```python
from build123d import *

# Parameters (mm, degrees)
F1_W     = 12
F1_H     = 14
F1_R     = 2.6
F2_DEPTH = 6
F3_DEPTH = 50
F4_R     = 11.5
F4_R_2   = 1.6
F5_DEPTH = 20.001
F7_R     = 5
F8_SIZE  = 2.5


with BuildPart() as f2:
    # F1 (on Top) → F2 (new body)
    with BuildSketch(Plane.XY):
        with Locations((-10, 30.4999971617)):
            Rectangle(F1_W, F1_H)
        with Locations((-10, 30.4999971617)):
            Circle(F1_R, mode=Mode.SUBTRACT)
        with BuildLine():
            Line((10, 33.0999971617), (10, 37.4999971617))
            Line((10, 37.4999971617), (4, 37.4999971617))
            Line((4, 37.4999971617), (4, 30.4999971617))
            Line((4, 30.4999971617), (7.4, 30.4999971617))
            ThreePointArc((7.4, 30.4999971617), (8.1615223689, 32.3384747928), (10, 33.0999971617))
        make_face()
        with BuildLine():
            Line((16, 30.4999971617), (16, 37.4999971617))
            Line((16, 37.4999971617), (10, 37.4999971617))
            Line((10, 37.4999971617), (10, 33.0999971617))
            ThreePointArc((10, 33.0999971617), (11.8384776311, 32.3384747928), (12.6, 30.4999971617))
            Line((12.6, 30.4999971617), (16, 30.4999971617))
        make_face()
        with BuildLine():
            Line((10, 23.4999971617), (16, 23.4999971617))
            Line((16, 23.4999971617), (16, 30.4999971617))
            Line((16, 30.4999971617), (12.6, 30.4999971617))
            ThreePointArc((12.6, 30.4999971617), (11.8384776311, 28.6615195306), (10, 27.8999971617))
            Line((10, 27.8999971617), (10, 23.4999971617))
        make_face()
        with BuildLine():
            Line((4, 23.4999971617), (10, 23.4999971617))
            Line((10, 23.4999971617), (10, 27.8999971617))
            ThreePointArc((10, 27.8999971617), (8.1615223689, 28.6615195306), (7.4, 30.4999971617))
            Line((7.4, 30.4999971617), (4, 30.4999971617))
            Line((4, 30.4999971617), (4, 23.4999971617))
        make_face()
        Polygon((-16, 37.4999971617), (-20, 23.4999971617), (-16, 23.4999971617), align=None)
        Polygon((-4, 37.4999971617), (-4, 23.4999971617), (4, 23.4999971617), (4, 30.4999971617), (4, 37.4999971617), align=None)
        Polygon((16, 23.4999971617), (20, 23.4999971617), (16, 37.4999971617), (16, 30.4999971617), align=None)
    extrude(amount=F2_DEPTH)

    # F1 (on Top) → F3 (join)
    with BuildSketch(Plane.XY):
        Polygon((-20, 23.4999971617), (-20, 17.4999971617), (20, 17.4999971617), (20, 23.4999971617), (16, 23.4999971617), (10, 23.4999971617), (4, 23.4999971617), (-4, 23.4999971617), (-16, 23.4999971617), align=None)
    extrude(amount=F3_DEPTH)

    # F4 (on face) → F5 (cut, through all)
    with BuildSketch(Plane.XZ.offset(-17.4999971617)):
        with Locations((0, 30)):
            Circle(F4_R)
        with Locations((-15.5, 45.5)):
            Circle(F4_R_2)
        with Locations((-15.5, 14.5)):
            Circle(F4_R_2)
        with Locations((15.5, 14.5)):
            Circle(F4_R_2)
        with Locations((15.5, 45.5)):
            Circle(F4_R_2)
    extrude(amount=-F5_DEPTH, mode=Mode.SUBTRACT)

    # F7
    f7_edges = [f2.edges().sort_by_distance(p)[0] for p in [
        (16, 37.499997, 3),
        (-16, 37.499997, 3),
    ]]
    fillet(f7_edges, radius=F7_R)

    # F8
    f8_edges = [f2.edges().sort_by_distance(p)[0] for p in [
        (-11.5, 23.499997, 30),
    ]]
    chamfer(f8_edges, length=F8_SIZE)


solid = f2.part
```
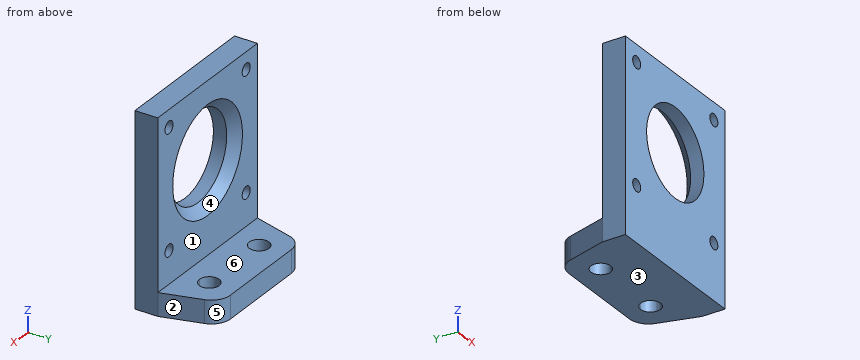
For this review, take the finished solid that the model builds, in its own axes (mm). Face numbers are marked on the shaded views. A direction names the side the tool comes from. Round coordinates to 2 decimals unless told otherwise and drop trailing zeros. Write each loop counter-clockwise with the first axis right and the second up, starting at its lowest first coordinate (ties: lowest second). Pieces come first, ordered by that corner, then holes. Notation, with made-up numbers: (-7, 42) - (16, 42) arc R28 ccw to (16, 70) - close; hole circle Ø7 at (53.25, 52). An arc over 180 degrees is marked (long way). Answer as a JSON object with one key per item and string values.
1. We need section D-D on z = 9.5. Give the boundary of the cut face in (x, y), then the cut area to 3 significant figures.
Response values:
{"outline": "(-20, 17.5) - (20, 17.5) - (20, 23.5) - (-20, 23.5) - close", "area": "240 mm2"}
2. Draft analysis for pull direction Z (two halves, no side actions). For the marked faces 3, 4, 5 and 6, state which applies: +Z half, -Z half, draft (parallel to the pull), parting line (faces both ways), or undercut.
Response values:
{"face 3": "-Z half", "face 4": "undercut", "face 5": "draft", "face 6": "+Z half"}
3. For pin 1 Ø5 at (x, y) = (-7, 21.5) entering from -Z; pin 2 Ø1.5 at (x, y) = (-5, 27.5) entering from +Z; pin 3 Ø3 at (x, z) = (13.5, 40) entering from +Y, all flat-tipped, find the tip position at first contact; note any pin that passes through.
Response values:
{"pin 1": "stops at z = 0", "pin 2": "stops at z = 6", "pin 3": "stops at y = 23.5"}
4. We need section B-B on y = 31.25. Give the boundary of the cut face in (x, z), then the cut area to 3 significant figures.
Response values:
{"outline": "(-17.79, 0) - (-12.49, 0) - (-12.49, 6) - (-17.79, 6) - close; (-7.51, 0) - (7.51, 0) - (7.51, 6) - (-7.51, 6) - close; (12.49, 0) - (17.79, 0) - (17.79, 6) - (12.49, 6) - close", "area": "154 mm2"}
5. Tool access review of the marked faces 1 and 2: name each direction out of +Z, -Z, +X, -X, +Y, -Y from which nothing blocks a thin tool from reaching the whole face with its end or side.
Response values:
{"face 1": "+Z, +X, -X, +Y", "face 2": "+Z, -Z, +X, +Y"}
6. To check wall thickness, follow line 1 along Z through (x, y) = (-15.5, 21.85); line 2 along Z through (x, y) = (16.5, 18.5); line 3 along Z through (x, y) = (0, 18.3). State the ranges of each line that lie inside material, in increasing order.
Response values:
{"line 1": "z = 0 to 12.9, 16.1 to 43.9, 47.1 to 50", "line 2": "z = 0 to 13.25, 15.75 to 44.25, 46.75 to 50", "line 3": "z = 0 to 18.5, 41.5 to 50"}
7. We need section C-C on x = 15.5. Give the boundary of the cut face in (y, z).
Response values:
{"outline": "(17.5, 0) - (36.28, 0) - (36.28, 6) - (23.5, 6) - (23.5, 12.9) - (17.5, 12.9) - close; (17.5, 16.1) - (23.5, 16.1) - (23.5, 43.9) - (17.5, 43.9) - close; (17.5, 47.1) - (23.5, 47.1) - (23.5, 50) - (17.5, 50) - close"}
8. We need section A-A on z = 14.5. Give the boundary of the cut face in (x, y).
Response values:
{"outline": "(-20, 17.5) - (-17.1, 17.5) - (-17.1, 23.5) - (-20, 23.5) - close; (-13.9, 17.5) - (13.9, 17.5) - (13.9, 23.5) - (-13.9, 23.5) - close; (17.1, 17.5) - (20, 17.5) - (20, 23.5) - (17.1, 23.5) - close"}
